Read the model definition and answer for the solid it produces. Units are mm, in the model's axes. Face numbers are marked on the shaded views. A direction names the side the tool comes from. Give positions to 0.01 mm unless a question says otherwise; leave off trailing zeros. Write each loop counter-clockwise with the first axis right and the second up, starting at its lowest first coordinate (ties: lowest second). Pieces come first, ordered by that corner, then holes.
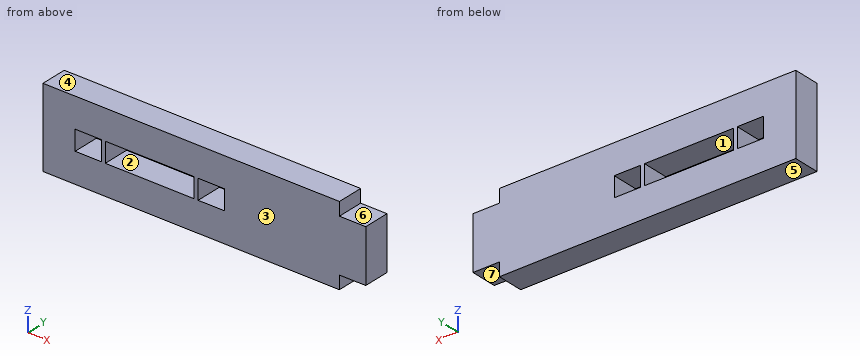
```python
from build123d import *

# Parameters (mm, degrees)
SKETCH1_W               = 45
SKETCH1_H               = 12
BOSS_EXTRUDE1_DEPTH     = 4
SKETCH2_W               = 8
SKETCH2_H               = 8
BOSS_EXTRUDE2_DEPTH     = 4
SKETCH4_W               = 13.5
SKETCH4_H               = 3
CUT_EXTRUDE2_DEPTH      = 5
SKETCH4_3_W             = 4
SKETCH4_3_H             = 3
CUT_EXTRUDE_THIN2_DEPTH = 4
LPATTERN1_COUNT         = 2
LPATTERN1_PITCH         = 18.67


with BuildPart() as part:
    # Sketch1 → Boss-Extrude1 (new body)
    with BuildSketch(Plane(origin=(0, 0, 0), x_dir=(1, 0, 0), z_dir=(0, 1, 0))):
        Rectangle(SKETCH1_W, SKETCH1_H)
    extrude(amount=BOSS_EXTRUDE1_DEPTH)

    # Sketch2 → Boss-Extrude2 (add)
    with BuildSketch(Plane(origin=(0, 0, 0), x_dir=(1, 0, 0), z_dir=(0, 1, 0))):
        with Locations((22.5, 0)):
            Rectangle(SKETCH2_W, SKETCH2_H)
    extrude(amount=BOSS_EXTRUDE2_DEPTH)

    # Sketch4 → Cut-Extrude2 (cut, through all)
    with BuildSketch(Plane(origin=(0, 0, 0), x_dir=(1, 0, 0), z_dir=(0, 1, 0))):
        with Locations((-6.29, 0)):
            Rectangle(SKETCH4_W, SKETCH4_H)
    extrude(amount=CUT_EXTRUDE2_DEPTH, mode=Mode.SUBTRACT)

    # Sketch4<3> → Cut-Extrude-Thin2 (cut)
    with BuildSketch(Plane(origin=(0, 0, 0), x_dir=(1, 0, 0), z_dir=(0, 1, 0))):
        with Locations((3.05, 0)):
            Rectangle(SKETCH4_3_W, SKETCH4_3_H)
    cut_extrude_thin2 = extrude(amount=CUT_EXTRUDE_THIN2_DEPTH, mode=Mode.SUBTRACT)

    # LPattern1: Cut-Extrude-Thin2 ×2
    with Locations(*[(-i * LPATTERN1_PITCH, 0, 0) for i in range(1, LPATTERN1_COUNT)]):
        add(cut_extrude_thin2, mode=Mode.SUBTRACT)


solid = part.part
```
Item 1: Find the intervals of material crossed by line 1 along X through (y, z) = (3.1, 1.25); line 2 along Z through (x, y) = (-17.5, 3.45); line 3 along X through (y, z) = (3.15, -4.25), in increasing order.
Result set:
line 1: x = -22.5 to -17.62, -13.62 to -13.04, 0.46 to 1.05, 5.05 to 26.5
line 2: z = -6 to -1.5, 1.5 to 6
line 3: x = -22.5 to 22.5
Item 2: Determine the mould class of the marked faces 1, 2, 3 and 4 for opening direction Z: pulls with the +Z half, pulls with the -Z half, needs draft (parallel to the pull), parting line crosses it, or undercut.
Result set:
face 1: undercut
face 2: undercut
face 3: needs draft
face 4: pulls with the +Z half
Item 3: Section B-B (y = 2.95) is taken. Write down the section's boundary in (x, z).
Result set:
outline: (-22.5, -6) - (22.5, -6) - (22.5, -4) - (26.5, -4) - (26.5, 4) - (22.5, 4) - (22.5, 6) - (-22.5, 6) - close; hole (-17.62, -1.5) - (-13.62, -1.5) - (-13.62, 1.5) - (-17.62, 1.5) - close; hole (-13.04, -1.5) - (0.46, -1.5) - (0.46, 1.5) - (-13.04, 1.5) - close; hole (1.05, -1.5) - (5.05, -1.5) - (5.05, 1.5) - (1.05, 1.5) - close
Item 4: Which of the six approach directions +Z, -Z, +X, -X, +Y, -Y give full straight-line access (tool end or side, diameter ignored) to the marked faces 5, 6 and 7?
Result set:
face 5: -Z, +X, -X, +Y, -Y
face 6: +Z, +X, +Y, -Y
face 7: -Z, +X, +Y, -Y
Item 5: Section A-A (x = 4.5) is taken. Write down the section's boundary in (y, z), and give its area (3 significant figures).
Result set:
outline: (0, -6) - (4, -6) - (4, -1.5) - (0, -1.5) - close; (0, 1.5) - (4, 1.5) - (4, 6) - (0, 6) - close
area: 36.0 mm2
Item 6: Section D-D (z = -5) is taken. Write down the section's boundary in (x, y), and give its area (3 significant figures).
Result set:
outline: (-22.5, 0) - (22.5, 0) - (22.5, 4) - (-22.5, 4) - close
area: 180 mm2
Item 7: This flat-tipped pin is pushed along its axis until it touches: pin 1 Ø1 at (y, z) = (1.5, -5) entering from +X. Where does it stop, or does it pass through?
Result set:
pin 1: stops at x = 22.5
Item 8: Section C-C (z = -0.5) is taken. Write down the section's boundary in (x, y), and give its area (3 significant figures).
Result set:
outline: (-22.5, 0) - (-17.62, 0) - (-17.62, 4) - (-22.5, 4) - close; (-13.62, 0) - (-13.04, 0) - (-13.04, 4) - (-13.62, 4) - close; (0.46, 0) - (1.05, 0) - (1.05, 4) - (0.46, 4) - close; (5.05, 0) - (26.5, 0) - (26.5, 4) - (5.05, 4) - close
area: 110 mm2
